Here's how the part is built. I have some questions about the finished solid (model axes, mm). Face numbers are marked on the shaded views. A direction names the side the tool comes from. Coordinates: 2 decimals unless noted, no trailing zeros. Loops run counter-clockwise (first coordinate to the right, second up) from the corner with the lowest first, then second, coordinate; pieces in that order, holes last. Notation, with made-up numbers: M 4.25,29.5 L 12.25,29.5 A26 ccw 12.25,58.5 Z; hole C -7,13 d3. An arc over 180 degrees is marked long. Use CSV: the item, a comma, the result in double quotes. Start each with the question number.
Q1. Please list where these lines run through material, in increasing order: probe 1 along Z at (x, y) = (-5, 33) (3 decimals); probe 2 along Y at (x, z) = (3, -13.5). Write a range as [from, to].
Q2. If we mould it in two halves opening along Z, with no side actions, what happens to the marked faces 3, 4 and 5? For each: +Z half, -Z half, draft (parallel to the pull), parting line (faces both ways), or undercut.
Q3. If we section it at A-A (y = 7): Please give me the cut outline in (x, z) (3 decimals).
Q4. Which directions (+Z, -Z, +X, -X, +Y, -Y) give clear straight access to the entire face, cutting with the end or side of a thin tool? Please do the marked faces 1 and 2.
Q5. For pin 1 Ø1 at (x, z) = (-0.5, 9) entering from +Y; pin 2 Ø4 at (y, z) = (4.5, -2.5) entering from +X, each with a flat end and sliding along its axis, tell me the tip position at first contact or that it passes through.
Q6. If we section it at C-C (z = 13.5): Please give me the cut outline in (x, y), and give its area (3 significant figures).
Q7. If we section it at B-B (x = -11): Please give me the cut outline in (y, z) (3 decimals), and give its area (3 significant figures).
Q8. If we section it at D-D (y = 12.5): Please give me the cut outline in (x, z) (3 decimals).
Autodesk Inventor part; units mm, degrees
ref_plane "YZ Plane" through (0, 0, 0) normal (1, 0, 0) x (0, 1, 0)
ref_plane "XZ Plane" through (0, 0, 0) normal (0, 1, 0) x (-1, 0, 0)
ref_plane "XY Plane" through (0, 0, 0) normal (0, 0, 1) x (1, 0, 0)
sketch "Sketch1" plane through (0, 0, 0) normal (0, 1, 0) x (-1, 0, 0)
  line L0 (15, -15.715) -> (-15, -15.715)
  line L1 (-15, -15.715) -> (-15, 15.715)
  line L2 (-15, 15.715) -> (15, 15.715)
  line L3 (15, 15.715) -> (15, -15.715)
  point P0 (0, 0)
  dimension "d0" = 30
  dimension "d1" = 15
  dimension "d2" = 31.43
  dimension "d3" = 15.715
extrude "Plate1" add sketch "Sketch1" along normal blind 1.5
sketch "Sketch2" plane through (15, 0, 17.215) normal (0, 0, -1) x (-1, 0, 0)
  line L0 (30, 0) -> (0, 0)
  line L1 (0, 0) -> (0, 40)
  line L2 (0, 40) -> (30, 40)
  line L3 (30, 40) -> (30, 0)
edge flange "Flange1" height 40 angle 90 thickness 1.5 bend radius 0.31 thickness toward (0, 0, -1) relief tear relief width 1.5 relief depth 0.75 edges at (0, 1.5, 15.715) wall of the first edge with corners at (-15, 0, 17.215) (15, 0, 17.215) (15, 40, 17.215) (-15, 40, 17.215)
bend "Bend1"
corner "Corner1"
sketch "Sketch3" plane through (-15, 0, -17.215) normal (0, 0, 1) x (1, 0, 0)
  line L0 (30, 0) -> (0, 0)
  line L1 (0, 0) -> (0, 40)
  line L2 (0, 40) -> (30, 40)
  line L3 (30, 40) -> (30, 0)
edge flange "Flange2" height 40 angle 90 thickness 1.5 bend radius 0.31 thickness toward (0, 0, 1) relief tear relief width 1.5 relief depth 0.75 edges at (0, 1.5, -15.715) wall of the first edge with corners at (15, 0, -17.215) (-15, 0, -17.215) (-15, 40, -17.215) (15, 40, -17.215)
bend "Bend2"
corner "Corner2"
sketch "Sketch4" plane through (-15, 40, 17.215) normal (0, 0, 1) x (1, 0, 0)
  circle A0 centre (15, -10) radius 10
  line L0 (0, 0) -> (30, 0)
  line L1 (30, 0) -> (30, -38.19)
  line L2 (5.3148, -7.5108) -> (0, -28.19)
  line L3 (0, -28.19) -> (0, -38.19)
  line L4 (0, -38.19) -> (30, -38.19)
  line L5 (30, -38.19) -> (30, -28.19)
  line L6 (30, -28.19) -> (24.6852, -7.5108)
  line L7 (0, -38.19) -> (30, -38.19)
  line L8 (0, -38.19) -> (0, 0)
  point P0 (15, -40)
  point P1 (0, -28.19)
  point P2 (15, 0)
  point P3 (30, -28.19)
  dimension "d25" = 10
  dimension "d26" = 15
  dimension "d27" = 20
  dimension "d29" = 30
  dimension "d30" = 0
  dimension "d31" = 10
  dimension "d32" = 10
  dimension "d33" = 0
extrude "Extrusion1" cut sketch "Sketch4" against normal blind 50 contours A0 L0 L1 L6 | L2 L8 L0 A0
equation "\"d4\" = Thickness"
equation "\"d5\" = BendReliefWidth"
equation "\"d6\" = BendReliefDepth"
equation "\"d7\" = MinimumRemnant"
equation "\"d8\" = TransitionRadius"
equation "\"d11\" = BendRadius"
equation "\"d12\" = CornerReliefSize"
equation "\"d13\" = GapSize"
equation "\"d14\" = JacobiRadiusSize"
equation "\"d15\" = BendReliefWidth"
equation "\"d16\" = BendReliefDepth"
equation "\"d17\" = MinimumRemnant"
equation "\"d18\" = TransitionRadius"
equation "\"d21\" = BendRadius"
equation "\"d22\" = CornerReliefSize"
equation "\"d23\" = GapSize"
equation "\"d24\" = JacobiRadiusSize"
equation "\"BendReliefWidth\" = Thickness"
equation "\"BendReliefDepth\" = 0.5 * Thickness"
equation "\"CornerReliefSize\" = 4 * Thickness"
equation "\"MinimumRemnant\" = 2 * Thickness"
equation "\"TransitionRadius\" = BendRadius"
equation "\"JacobiRadiusSize\" = BendRadius"
equation "\"GapSize\" = Thickness"
properties part number "axis_12_bottom_frame(top)" material "Aluminum 6061-AHC"
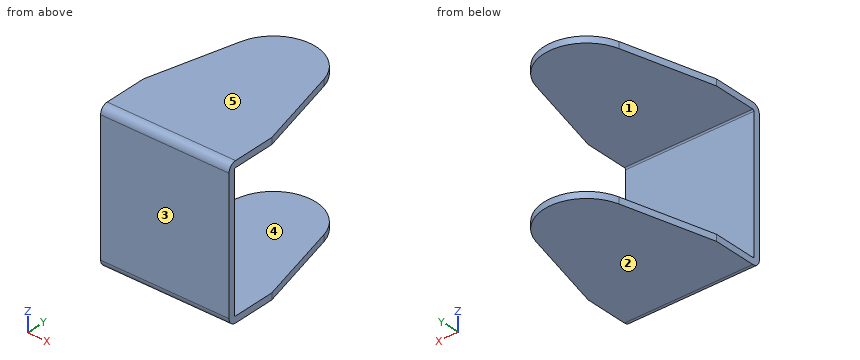
Results below:
1,probe 1,"[-17.215, -15.715], [15.715, 17.215]"
1,probe 2,"[0, 1.5]"
2,face 3,"draft"
2,face 4,"undercut"
2,face 5,"+Z half"
3,outline,"M -15,-17.215 L 15,-17.215 L 15,-15.715 L -15,-15.715 Z; M -15,15.715 L 15,15.715 L 15,17.215 L -15,17.215 Z"
4,face 1,"+X, -X, +Y"
4,face 2,"-Z, +X, -X, +Y, -Y"
5,pin 1,"y = 1.5"
5,pin 2,"through"
6,outline,"M -15,0 L 15,0 L 15,1.5 L -15,1.5 Z"
6,area,"45.0 mm^2"
7,outline,"M 0,-15.405 A1.81 ccw 1.81,-17.215 L 27.373,-17.215 L 27.373,-15.715 L 1.81,-15.715 A0.31 cw 1.5,-15.405 L 1.5,15.405 A0.31 cw 1.81,15.715 L 27.373,15.715 L 27.373,17.215 L 1.81,17.215 A1.81 ccw 0,15.405 Z"
7,area,"128 mm^2"
8,outline,"M -14.823,-17.215 L 14.823,-17.215 L 14.823,-15.715 L -14.823,-15.715 Z; M -14.823,15.715 L 14.823,15.715 L 14.823,17.215 L -14.823,17.215 Z"
